For this review, take the finished solid that the model builds, in its own axes (mm). A direction names the side the tool comes from. Coordinates: 2 decimals unless noted, no trailing zeros. Loops run counter-clockwise (first coordinate to the right, second up) from the corner with the lowest first, then second, coordinate; pieces in that order, holes last. Notation, with made-up numbers: M 2.25,33 L 32.25,33 A22 cw 32.25,44 Z; hole C 23.25,24 d7. An arc over 180 degrees is marked long. Put each result on its own line as item: value.
```python
from build123d import *

# Parameters (mm, degrees)
F1_DEPTH = 44.45
F2_SIZE  = 12.7
F3_W     = 15.875
F3_H     = 6.35
F4_DEPTH = 241.3


with BuildPart() as f1:
    # F0 (on Front) → F1 (new body, symmetric)
    with BuildSketch(Plane.XZ):
        Polygon((228.6, -20.6375), (228.6, 20.6375), (146.05, 20.6375), (146.05, 65.0875), (-139.7, 65.0875), (-139.7, 20.6375), (-228.6, 20.6375), (-228.6, -20.6375), align=None)
    extrude(amount=F1_DEPTH, both=True)

    # F2
    f2_edges = [f1.edges().sort_by_distance(p)[0] for p in [
        (146.05, 0, 65.0875),
        (-139.7, 0, 65.0875),
        (-228.6, 0, 20.6375),
        (228.6, 0, 20.6375),
    ]]
    chamfer(f2_edges, length=F2_SIZE)

    # F3 (on Right) → F4 (cut, symmetric)
    with BuildSketch(Plane.YZ):
        with Locations((-23.8125, -17.4625)):
            Rectangle(F3_W, F3_H)
        with Locations((23.8125, -17.4625)):
            Rectangle(F3_W, F3_H)
    extrude(amount=F4_DEPTH, both=True, mode=Mode.SUBTRACT)


solid = f1.part
```
(1) Add section C-C (z = 38). Write out the cut boundary in (x, y).
Determined:
outline: M -139.7,-44.45 L 146.05,-44.45 L 146.05,44.45 L -139.7,44.45 Z
(2) Add section B-B (y = 37). Write out the cut boundary in (x, z).
Determined:
outline: M -228.6,-20.64 L 228.6,-20.64 L 228.6,7.94 L 215.9,20.64 L 146.05,20.64 L 146.05,52.39 L 133.35,65.09 L -127,65.09 L -139.7,52.39 L -139.7,20.64 L -215.9,20.64 L -228.6,7.94 Z
(3) Draft analysis for pull direction Y (two halves, no side actions). For faces 4 (the flat face through (3, 24, -14.287)), 5 (the flat face through (-177, -1, 20.638)), 6 (the flat face through (-3, 44.45, 13)), 7 (the flat face through (-3, -24, -14.287)), state which applies: +Y half, -Y half, draft (parallel to the pull), parting line (faces both ways), or undercut.
Determined:
face 4: undercut
face 5: draft
face 6: +Y half
face 7: undercut
(4) For pin 1 (16 mm diameter, centred on y = 0.5, z = 34.5, fed in from +X); pin 2 (10 mm diameter, centred on y = -34, z = 22, fed in from +X); pin 3 (1.5 mm diameter, centred on y = 19, z = 55, fed in from -X), all flat-tipped, find the tip position at first contact; note any pin that passes through.
Determined:
pin 1: stops at x = 146.05
pin 2: stops at x = 219.54
pin 3: stops at x = -137.84
(5) Wall thickness on line 1 along Y through (x, z) = (193.5, -17) (3 decimals); line 2 along Z through (x, y) = (77, -28.5); line 3 along X through (y, z) = (1, 31.5): over which ranges is each line inside the solid? List them lowest first. Write a range as [from, to].
Determined:
line 1: y = [-44.45, -31.75], [-15.875, 15.875], [31.75, 44.45]
line 2: z = [-14.29, 65.09]
line 3: x = [-139.7, 146.05]
(6) Tool access review of faces 1 (the flat face through (-3, 0, -20.638)), 2 (the flat face through (146.05, -1, 36)), 3 (the flat face through (-139.7, -1, 37)): name each direction out of +Z, -Z, +X, -X, +Y, -Y from which nothing blocks a thin tool from reaching the whole face with its end or side.
Determined:
face 1: -Z, +X, -X, +Y, -Y
face 2: +Z, +X, +Y, -Y
face 3: +Z, -X, +Y, -Y
